Check sheet for the modelled part. Datum: model origin and axes. Units: mm. Give positions to 0.01 mm unless a question says otherwise; leave off trailing zeros. Loops run counter-clockwise (first coordinate to the right, second up) from the corner with the lowest first, then second, coordinate; pieces in that order, holes last.
```python
from build123d import *

# Parameters (mm, degrees)
SKETCH4_R           = 2.54
SKETCH4_R_2         = 3.175
SKETCH4_R_3         = 1.7272
SKETCH4_W           = 6.35
SKETCH4_H           = 63.5
BOSS_EXTRUDE4_DEPTH = 6.35
FILLET1_R           = 6.35
FILLET2_R           = 3.175


with BuildPart() as part:
    # Sketch4 → Boss-Extrude4 (new body)
    with BuildSketch(Plane.XY):
        Polygon((58.871875, 44.45), (96.971875, 44.45), (96.971875, -44.45), (58.871875, -44.45), (58.871875, -9.525), (-65.221875, -9.525), (-65.221875, -44.45), (-115.921875, -44.45), (-115.921875, 44.45), (-65.221875, 44.45), (-65.221875, 9.525), (58.871875, 9.525), align=None)
        with Locations((-109.571875, 38.1)):
            Circle(SKETCH4_R, mode=Mode.SUBTRACT)
        with Locations((84.271875, 38.1)):
            Circle(SKETCH4_R_2, mode=Mode.SUBTRACT)
        with Locations((46.171875, 0)):
            Circle(SKETCH4_R_3, mode=Mode.SUBTRACT)
        with Locations((20.771875, 0)):
            Circle(SKETCH4_R_3, mode=Mode.SUBTRACT)
        with Locations((-4.628125, 0)):
            Circle(SKETCH4_R_3, mode=Mode.SUBTRACT)
        with Locations((-30.028125, 0)):
            Circle(SKETCH4_R_3, mode=Mode.SUBTRACT)
        with Locations((71.571875, 38.1)):
            Circle(SKETCH4_R, mode=Mode.SUBTRACT)
        with Locations((-71.571875, 38.1)):
            Circle(SKETCH4_R, mode=Mode.SUBTRACT)
        with Locations(Location((84.271875, -38.1, 0), (0, 0, 180))):
            Circle(SKETCH4_R_2, mode=Mode.SUBTRACT)
        with Locations(Location((71.571875, -38.1, 0), (0, 0, 180))):
            Circle(SKETCH4_R, mode=Mode.SUBTRACT)
        with Locations(Location((-71.571875, -38.1, 0), (0, 0, 180))):
            Circle(SKETCH4_R, mode=Mode.SUBTRACT)
        with Locations(Location((-109.571875, -38.1, 0), (0, 0, 180))):
            Circle(SKETCH4_R, mode=Mode.SUBTRACT)
        with Locations((84.271875, 0)):
            Circle(SKETCH4_R_2, mode=Mode.SUBTRACT)
        with Locations((-55.428125, 0)):
            Circle(SKETCH4_R_3, mode=Mode.SUBTRACT)
        with Locations((68, 0)):
            Rectangle(SKETCH4_W, SKETCH4_H, mode=Mode.SUBTRACT)
    extrude(amount=BOSS_EXTRUDE4_DEPTH)

    # Fillet1
    fillet1_edges = [part.edges().sort_by_distance(p)[0] for p in [
        (58.871875, -9.525, 3.175),
        (-65.221875, -9.525, 3.175),
        (-65.221875, -44.45, 3.175),
        (-115.921875, -44.45, 3.175),
        (-115.921875, 44.45, 3.175),
        (-65.221875, 44.45, 3.175),
        (-65.221875, 9.525, 3.175),
        (58.871875, 9.525, 3.175),
        (58.871875, 44.45, 3.175),
        (96.971875, 44.45, 3.175),
        (96.971875, -44.45, 3.175),
        (58.871875, -44.45, 3.175),
    ]]
    fillet(fillet1_edges, radius=FILLET1_R)

    # Fillet2
    fillet2_edges = [part.edges().sort_by_distance(p)[0] for p in [
        (71.175, 31.75, 3.175),
        (64.825, 31.75, 3.175),
        (71.175, -31.75, 3.175),
        (64.825, -31.75, 3.175),
    ]]
    fillet(fillet2_edges, radius=FILLET2_R - 0.0001)  # a hair under: the kernel refuses the full size


solid = part.part
```
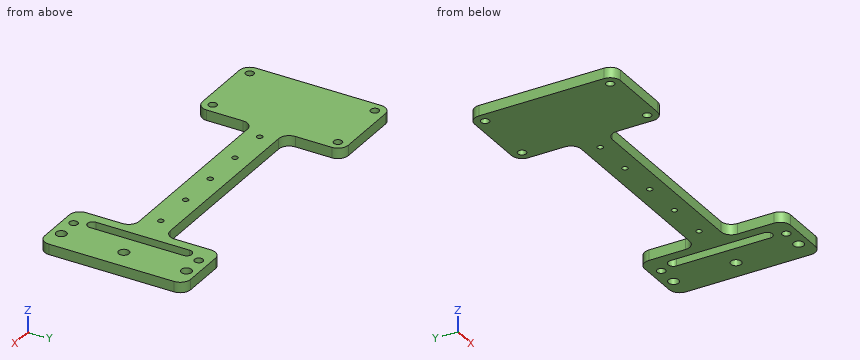
(1) Section check A-A on y = 24. Record the boundary of the cut face in (x, z) (3 decimals), plus the area to 3 significant figures.
(2) Section check C-C on x = -34. Record the boundary of the cut face in (y, z) (3 decimals), plus the area to 3 significant figures.
(3) Section check B-B on z = 4. Give the number of separate pieces and of enclosed holes in the cut face, plus the area to 3 significant figures.
(4) Material ranges on line 1 (X direction, y = -38.1, z = 2); line 2 (X direction, y = 17.5, z = 1.5) (3 decimals); line 3 (X direction, y = -8, z = 4.75) (3 decimals), recorded low to high.
Computed values:
1. outline: (-115.922, 0) - (-65.222, 0) - (-65.222, 6.35) - (-115.922, 6.35) - close; (58.872, 0) - (64.825, 0) - (64.825, 6.35) - (58.872, 6.35) - close; (71.175, 0) - (96.972, 0) - (96.972, 6.35) - (71.175, 6.35) - close
1. area: 524 mm2
2. outline: (-9.525, 0) - (9.525, 0) - (9.525, 6.35) - (-9.525, 6.35) - close
2. area: 121 mm2
3. separate pieces: 1
3. enclosed holes: 15
3. area: 9,570 mm2
4. line 1: x = -115.92 to -112.11, -107.03 to -74.11, -69.03 to -65.22, 58.87 to 69.03, 74.11 to 81.1, 87.45 to 96.97
4. line 2: x = -115.922 to -65.222, 58.872 to 64.825, 71.175 to 96.972
4. line 3: x = -115.922 to 64.825, 71.175 to 96.972
